```python
from build123d import *

# Parameters (mm, degrees)
F1_DEPTH = 12.5
F2_W     = 19.5208349061
F2_H     = 13
F3_DEPTH = 12.001
F4_W     = 21.5208349061
F4_H     = 13
F5_DEPTH = 12.001
F6_R     = 4
F7_DEPTH = 25.001


with BuildPart() as f1:
    # F0 (on Front) → F1 (new body, symmetric)
    with BuildSketch(Plane.XZ):
        with BuildLine():
            ThreePointArc((137.9791650939, 12), (138.369730009, 6.0056487784), (138.5, 0))
            Line((138.5, 0), (163.5, 0))
            Line((163.5, 0), (163.5, 12))
            Line((163.5, 12), (137.9791650939, 12))
        make_face()
        with BuildLine():
            Line((-163.5, 0), (-138.5, 0))
            ThreePointArc((-138.5, 0), (-138.369730009, 6.0056487784), (-137.9791650939, 12))
            Line((-137.9791650939, 12), (-163.5, 12))
            Line((-163.5, 12), (-163.5, 0))
        make_face()
        with BuildLine():
            ThreePointArc((-113.5, 0), (0, 113.5), (113.5, 0))
            Line((113.5, 0), (138.5, 0))
            ThreePointArc((138.5, 0), (138.369730009, 6.0056487784), (137.9791650939, 12))
            ThreePointArc((137.9791650939, 12), (0, 138.5), (-137.9791650939, 12))
            ThreePointArc((-137.9791650939, 12), (-138.369730009, 6.0056487784), (-138.5, 0))
            Line((-138.5, 0), (-113.5, 0))
        make_face()
    extrude(amount=F1_DEPTH, both=True)

    # F2 (on face) → F3 (cut, through all)
    with BuildSketch(Plane.XY.offset(12)):
        with Locations((153.7395825469, 0)):
            Rectangle(F2_W, F2_H)
    extrude(amount=-F3_DEPTH, mode=Mode.SUBTRACT)

    # F4 (on face) → F5 (cut, through all)
    with BuildSketch(Plane.XY.offset(12)):
        with Locations((-152.7395825469, 0)):
            Rectangle(F4_W, F4_H)
    extrude(amount=-F5_DEPTH, mode=Mode.SUBTRACT)

    # F6 (on face) → F7 (cut, through all)
    with BuildSketch(Plane.XZ.offset(12.5)):
        with Locations((155.5, 6)):
            Circle(F6_R)
    extrude(amount=-F7_DEPTH, mode=Mode.SUBTRACT)


solid = f1.part
```
Check sheet for the modelled part. Datum: model origin and axes. Units: mm. A direction names the side the tool comes from. Coordinates: 2 decimals unless noted, no trailing zeros. Loops run counter-clockwise (first coordinate to the right, second up) from the corner with the lowest first, then second, coordinate; pieces in that order, holes last.
1) Material ranges on probe 1 along Z at (x, y) = (155.5, -9); probe 2 along X at (y, z) = (3, 23); probe 3 along X at (y, z) = (2.5, 17.5), recorded low to high.
2) Sectioned sample at C-C (z = 6). Record the boundary of the cut face in (x, y), and give its area (3 significant figures).
3) Sectioned sample at A-A (x = 155.5). Record the boundary of the cut face in (y, z).
4) Sectioned sample at D-D (x = 0). Record the boundary of the cut face in (y, z), and give its area (3 significant figures).
5) Sectioned sample at B-B (z = 48.5). Record the boundary of the cut face in (x, y).
6) Gauge pin test, flat ends, axial feed: pin 1 (3 mm diameter, centred on y = -5.5, z = 45, fed in from -X); pin 2 (8 mm diameter, centred on y = 2, z = 90, fed in from +X); pin 3 (6 mm diameter, centred on x = -57.5, y = 3.5, fed in from -Z). Record the tip position at first contact, or that the pin passes through.
7) Access from +Z, -Z, +X, -X, +Y, -Y to the whole of each face (thin tool, end or side, straight path). Record for faces 4 (the face through (-151, -9, 12)), 5 (the face through (143.979, 0, 6)), 6 (the face through (-2.496, -0.175, 113.473)), 7 (the face through (-153, -6.5, 6)), 8 (the face through (142, 0, 12)).
8) Release check for a two-part mould opening along X. For faces 1 (the face through (-141.979, 0, 6)), 2 (the face through (151, -6.5, 6)), 3 (the face through (159.315, -9.542, 7.201)) record: released by +X, released by -X, zero draft, split by the parting line, or undercut.
Check sheet entries:
1. probe 1: z = 0 to 2, 10 to 12
1. probe 2: x = -136.58 to -111.15, 111.15 to 136.58
1. probe 3: x = -137.39 to -112.14, 112.14 to 137.39
2. outline: (-163.5, -12.5) - (-113.34, -12.5) - (-113.34, 12.5) - (-163.5, 12.5) - (-163.5, 6.5) - (-141.98, 6.5) - (-141.98, -6.5) - (-163.5, -6.5) - close; (113.34, -12.5) - (151.5, -12.5) - (151.5, -6.5) - (143.98, -6.5) - (143.98, 6.5) - (151.5, 6.5) - (151.5, 12.5) - (113.34, 12.5) - close; (159.5, -12.5) - (163.5, -12.5) - (163.5, -6.5) - (159.5, -6.5) - close; (159.5, 6.5) - (163.5, 6.5) - (163.5, 12.5) - (159.5, 12.5) - close
2. area: 1,880 mm2
3. outline: (-12.5, 0) - (-6.5, 0) - (-6.5, 2) - (-12.5, 2) - close; (-12.5, 10) - (-6.5, 10) - (-6.5, 12) - (-12.5, 12) - close; (6.5, 0) - (12.5, 0) - (12.5, 2) - (6.5, 2) - close; (6.5, 10) - (12.5, 10) - (12.5, 12) - (6.5, 12) - close
4. outline: (-12.5, 113.5) - (12.5, 113.5) - (12.5, 138.5) - (-12.5, 138.5) - close
4. area: 625 mm2
5. outline: (-129.73, -12.5) - (-102.62, -12.5) - (-102.62, 12.5) - (-129.73, 12.5) - close; (102.62, -12.5) - (129.73, -12.5) - (129.73, 12.5) - (102.62, 12.5) - close
6. pin 1: stops at x = -131.49
6. pin 2: stops at x = 108.56
6. pin 3: stops at z = 96.03
7. face 4: +Z, -X, +Y, -Y
7. face 5: +Z, -Z, +X
7. face 6: -Z, +Y, -Y
7. face 7: +Z, -Z, -X
7. face 8: +Z, +X, +Y, -Y
8. face 1: released by -X
8. face 2: zero draft
8. face 3: undercut
